Part model, mm, in its own coordinate system. Coordinates: 2 decimals unless noted, no trailing zeros. Loops run counter-clockwise (first coordinate to the right, second up) from the corner with the lowest first, then second, coordinate; pieces in that order, holes last. Notation, with made-up numbers: M 53,-26.5 L 89,-26.5 A23 cw 89,12.5 Z; hole C 10,14 d9. An arc over 180 degrees is marked long. Use CSV: the item, a comma, the result in double quotes. Start each with the question number.
from build123d import *

# Parameters (mm, degrees)
SKETCH1_W             = 33.29
SKETCH1_H             = 58.96
SKETCH1_R             = 1.8288
BOSS_EXTRUDE1_DEPTH   = 6.35
CUT_EXTRUDE1_DEPTH    = 169.208568246
FILLET1_R             = 2.5
FILLET2_R             = 2.5
F_6_32_TAPPED_HOLE1_D = 2.7051


with BuildPart() as part:
    # Sketch1 → Boss-Extrude1 (new body)
    # profile 1 of 2: a face of its own
    with BuildSketch(Plane(origin=(0, 0, 0), x_dir=(0, 0, -1), z_dir=(1, 0, 0))):
        with BuildLine():
            ThreePointArc((-7.249242854, 160.438616345), (0, 167.2625), (7.249242854, 160.438616345))
            Line((7.249242854, 160.438616345), (16.645, 5.15))
            Line((16.645, 5.15), (-16.645, 5.15))
            Line((-16.645, 5.15), (-7.249242854, 160.438616345))
        make_face()
    # profile 2 of 2: a face of its own
    with BuildSketch(Plane(origin=(0, 0, 0), x_dir=(0, 0, -1), z_dir=(1, 0, 0))):
        with Locations((0, -24.33)):
            Rectangle(SKETCH1_W, SKETCH1_H)
        with Locations((13.4747, -50)):
            Circle(SKETCH1_R, mode=Mode.SUBTRACT)
        with Locations((-13.4747, -50)):
            Circle(SKETCH1_R, mode=Mode.SUBTRACT)
        with Locations((13.4747, 0)):
            Circle(SKETCH1_R, mode=Mode.SUBTRACT)
        with Locations((-13.4747, 0)):
            Circle(SKETCH1_R, mode=Mode.SUBTRACT)
    extrude(amount=BOSS_EXTRUDE1_DEPTH)

    # Sketch2 → Cut-Extrude1 (cut, through all)
    with BuildSketch(Plane(origin=(6.35, 0, 0), x_dir=(0, 0, -1), z_dir=(1, 0, 0))):
        Polygon((11.645, -5.219501679), (1.407493202, -25), (11.645, -44.780498321), align=None)
        Polygon((0, -27.719501679), (-10.237506798, -47.5), (10.237506798, -47.5), align=None)
        Polygon((-11.645, -5.219501679), (-11.645, -44.780498321), (-1.407493202, -25), align=None)
        Polygon((-10.237506798, -2.5), (0, -22.280498321), (10.237506798, -2.5), align=None)
    extrude(amount=-CUT_EXTRUDE1_DEPTH, mode=Mode.SUBTRACT)

    # Fillet1
    fillet1_edges = [part.edges().sort_by_distance(p)[0] for p in [
        (3.175, -44.780498321, 11.645),
        (3.175, -5.219501679, 11.645),
        (3.175, -25, 1.407493202),
        (3.175, -47.5, -10.237506798),
        (3.175, -47.5, 10.237506798),
        (3.175, -27.719501679, 0),
        (3.175, -22.280498321, 0),
        (3.175, -2.5, 10.237506798),
        (3.175, -2.5, -10.237506798),
        (3.175, -25, -1.407493202),
        (3.175, -5.219501679, -11.645),
        (3.175, -44.780498321, -11.645),
    ]]
    fillet(fillet1_edges, radius=FILLET1_R)

    # Fillet2
    # the kernel refuses this fillet: 2.5 mm, written as the material it takes off along each edge
    with BuildSketch(Plane(origin=(-0.188905784, 5.15, -16.645), x_dir=(0, 0.9981745753787551, 0.06039467747609822), z_dir=(1, 0, 0))) as fillet2_piece_1:
        with BuildLine():
            CenterArc((FILLET2_R * 0.0302249253995, FILLET2_R), FILLET2_R, 266.537532795, 3.462467205)
            Line((-FILLET2_R * 0.0301697520766, FILLET2_R * 0.00182542462124), (0, 0))
            Line((0, 0), (FILLET2_R * 0.0302249253996, 0))
        make_face()
    extrude(amount=6.727811567, mode=Mode.SUBTRACT)
    with BuildSketch(Plane(origin=(-6.25, -53.81, -16.645), x_dir=(0, 1, 0), z_dir=(1, 0, 0))) as fillet2_piece_2:
        with BuildLine():
            CenterArc((FILLET2_R, FILLET2_R), FILLET2_R, 180, 90)
            Line((0, FILLET2_R), (0, 0))
            Line((0, 0), (FILLET2_R, 0))
        make_face()
    extrude(amount=18.85, mode=Mode.SUBTRACT)
    with BuildSketch(Plane(origin=(-6.25, -53.81, 16.645), x_dir=(0, 1, 0), z_dir=(1, 0, 0))) as fillet2_piece_3:
        with BuildLine():
            CenterArc((FILLET2_R, -FILLET2_R), FILLET2_R, 90, 90)
            Line((0, -FILLET2_R), (0, 0))
            Line((0, 0), (FILLET2_R, 0))
        make_face()
    extrude(amount=18.85, mode=Mode.SUBTRACT)
    with BuildSketch(Plane(origin=(-0.188905784, 5.15, 16.645), x_dir=(0, 0.9981745753787543, -0.06039467747611318), z_dir=(1, 0, 0))) as fillet2_piece_4:
        with BuildLine():
            CenterArc((FILLET2_R * 0.0302249253995, -FILLET2_R), FILLET2_R, 90, 3.462467205)
            Line((-FILLET2_R * 0.0301697520766, -FILLET2_R * 0.00182542462124), (0, 0))
            Line((0, 0), (FILLET2_R * 0.0302249253996, 0))
        make_face()
    extrude(amount=6.727811567, mode=Mode.SUBTRACT)

    # #6-32 Tapped Hole1 (through all)
    with Locations(Plane(origin=(6.35, 0, 0), x_dir=(0, 0, -1), z_dir=(1, 0, 0))):
        with Locations((0, 160.438616345)):
            Hole(F_6_32_TAPPED_HOLE1_D / 2)


solid = part.part
1. Pin check, flat tips, straight feed: pin 1 (1.9 mm diameter, centred on x = 4.5, z = 2.5, fed in from +Y); pin 2 (3 mm diameter, centred on y = -50, z = -13.47, fed in from -X); pin 3 (2 mm diameter, centred on x = 4.5, y = 91, fed in from +Z). Stop position of each tip, or through.
2. Two-plate mould, pull along Z, no slides. Class faces 1 (the face through (3.13, -46.27, 8.28)), 2 (the face through (3, -53.81, 0)): pulls with the +Z half, pulls with the -Z half, needs draft (parallel to the pull), parting line crosses it, or undercut.
3. Wall check: probe 1 along Y at (x, z) = (3.5, 0); probe 2 along Y at (x, z) = (0.75, 2); probe 3 along Z at (x, y) = (3.25, -32) (3 decimals). Give the ranges that are in metal, low to high.
4. Slice it at A-A, the plane y = 0. State how many separate pieces and enclosed holes the cut face has, and give its area (3 significant figures).
5. Slice it at D-D, the plane y = 123. List the corners of the cut face in (x, z), and give its area (3 significant figures).
6. Slice it at B-B, the plane y = -39. List the corners of the cut face in (x, z) (3 decimals), and give its area (3 significant figures).
Found:
1,pin 1,"y = 167.1"
1,pin 2,"through"
1,pin 3,"z = 11.51"
2,face 1,"undercut"
2,face 2,"needs draft"
3,probe 1,"-53.81 to -47.5, -30.66 to -19.34, -2.5 to 159.09, 161.79 to 167.26"
3,probe 2,"-53.81 to -47.5, -31.66 to -26.14, -23.86 to -18.34, -2.5 to 166.98"
3,probe 3,"-16.645 to -11.645, -5.03 to -2.215, 2.215 to 5.03, 11.645 to 16.645"
4,separate pieces,"3"
4,enclosed holes,"0"
4,area,"165 mm^2"
5,outline,"M 0,-9.51 L 6.35,-9.51 L 6.35,9.51 L 0,9.51 Z"
5,area,"121 mm^2"
6,outline,"M 0,-16.645 L 6.35,-16.645 L 6.35,-5.838 L 0,-5.838 Z; M 0,5.838 L 6.35,5.838 L 6.35,16.645 L 0,16.645 Z"
6,area,"137 mm^2"
